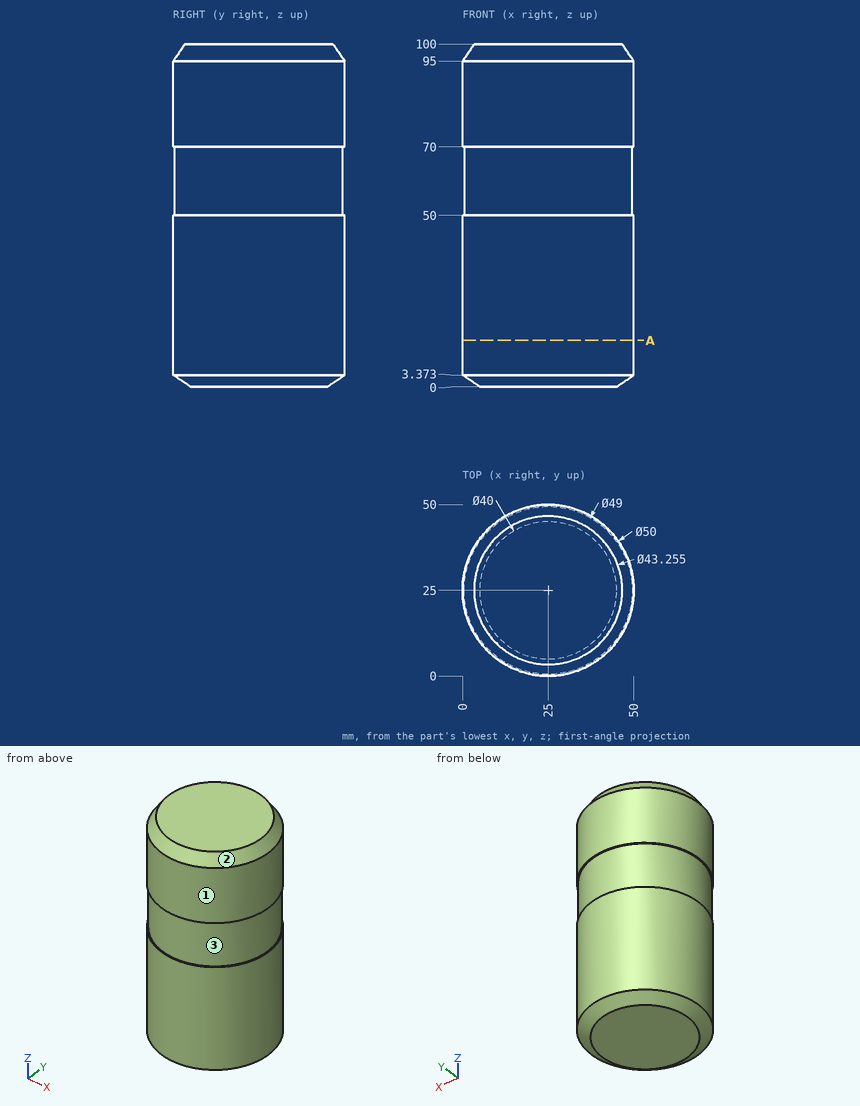
Answer from the drawing. Dimensions are ordinates in mm from the lowest x, y and z of the part. Round coordinates to 2 decimals unless told otherwise and drop trailing zeros. Loops run counter-clockwise (first coordinate to the right, second up) from the corner with the lowest first, then second, coordinate; pieces in that order, holes last.
Q1. Consider probe 1 along X at (y, z) = (26, 31); probe 2 along X at (y, z) = (24, 51.5); probe 3 along Y at (x, z) = (20, 31) (1 decimal). Determine where each line is inside the solid, lowest interval first.
Q2. Determine the mould class of the marked faces 1, 2 and 3 for opening direction Z: released by +Z, released by -Z, zero draft, split by the parting line, or undercut.
Q3. Each of these flat-tipped pins is pushed along its axis until it touches: pin 1 (8 mm diameter, centred on y = 25.5, z = 20.5, fed in from -X); pin 2 (3 mm diameter, centred on y = 42, z = 88, fed in from -X) (1 decimal); pin 3 (3 mm diameter, centred on y = 21.5, z = 65.5, fed in from -X); pin 4 (3 mm diameter, centred on x = 11.5, z = 37, fed in from +Y). Where does it stop, or does it pass through?
Q4. Section A-A on z = 13.5 is taken. Write down the section's boundary in (x, y).
Output:
1. probe 1: x = 0.02 to 49.98
1. probe 2: x = 0.52 to 49.48
1. probe 3: y = 0.5 to 49.5
2. face 1: zero draft
2. face 2: released by +Z
2. face 3: undercut
3. pin 1: stops at x = 0
3. pin 2: stops at x = 5.4
3. pin 3: stops at x = 0.58
3. pin 4: stops at y = 46.93
4. outline: circle Ø50 at (25, 25)
